Read the model definition and answer for the solid it produces. Units are mm, in the model's axes. Face numbers are marked on the shaded views. A direction names the side the tool comes from. Give positions to 0.01 mm unless a question says otherwise; leave off trailing zeros. Loops run counter-clockwise (first coordinate to the right, second up) from the corner with the lowest first, then second, coordinate; pieces in that order, holes last. Notation, with made-up numbers: (89, 34) - (140, 34) arc R23 ccw to (140, 58) - close; hole circle Ø1 at (-38.75, 37.25). An arc over 180 degrees is marked (long way). Put each result on its own line as item: value. Start each with the question number.
1. For the marked faces 1, 2, 3 and 4, determine the directions among +Z, -Z, +X, -X, +Y, -Y from which every point of the face is accessible in a straight line to the end or side of a thin tool.
2. A cutting plane is placed at A-A, the plane z = -4.5. Determine the outline of the cut face in (x, y).
3. A cutting plane is placed at B-B, the plane x = -27. Determine the outline of the cut face in (y, z).
4. A cutting plane is placed at D-D, the plane z = -10.5. Determine the outline of the cut face in (x, y), plus the area to 3 significant figures.
5. Consider L1, parallel to Z at x = -22.5, y = 1.7; L2, parallel to Y at x = -27, z = 6.05; L3, parallel to Z at x = -10, y = 3.9. Determine where each line is inside the solid, lowest interval first. Write a range as from..to.
6. Given pin 1 Ø1.9 at (x, y) = (-4, 3) entering from -Z; pin 2 Ø3 at (y, z) = (5, -3.5) entering from -X; pin 3 Ø2.5 at (y, z) = (2, 6) entering from -X; pin 4 Ø1.5 at (y, z) = (2.5, -10) entering from -X, each flat-ended and moving along its own axis, determine where each tip first touches the part or whether it passes through.
7. A cutting plane is placed at C-C, the plane x = -4. Determine the outline of the cut face in (y, z), plus the area to 3 significant figures.
8. For a pull along Z with two mould halves and no side action, classify the marked faces 5, 6, 7 and 8 as released by +Z, released by -Z, zero draft, split by the parting line, or undercut.
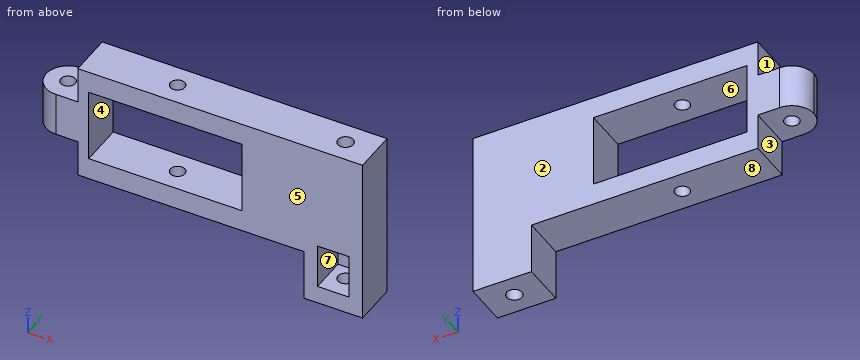
Autodesk Inventor part; units mm, degrees
ref_plane "Pracovní rovina1" through (0, 0, 0) normal (0, 0, -1) x (-1, 0, 0)
ref_plane "YZ Plane" through (0, 0, 0) normal (1, 0, 0) x (0, 1, 0)
ref_plane "XZ Plane" through (0, 0, 0) normal (0, 1, 0) x (-1, 0, 0)
sketch "Sketch1" plane through (0, 0, 0) normal (0, 1, 0) x (-1, 0, 0)
  line L0 (0, 0) -> (18.1846, 0) construction
  line L1 (0, 0) -> (0, 15)
  line L2 (0, 15) -> (8, 15)
  line L3 (8, 15) -> (8, 8)
  line L4 (8, 8) -> (39, 8)
  line L5 (39, 8) -> (39, 3)
  line L6 (39, 3) -> (45, 3)
  line L7 (45, 3) -> (45, 0)
  line L8 (0, 0) -> (0, -15)
  line L9 (0, -15) -> (8, -15)
  line L10 (8, -15) -> (8, -8)
  line L11 (8, -8) -> (39, -8)
  line L12 (39, -8) -> (39, -3)
  line L13 (39, -3) -> (45, -3)
  line L14 (45, -3) -> (45, 0)
  point P0 (45, 1.5)
  dimension "d0" = 6
  dimension "d1" = 45
  dimension "d2" = 8
  dimension "d3" = 8
  dimension "d4" = 15
  dimension "d5" = 3
extrude "Extrusion1" add sketch "Sketch1" along normal blind 6
sketch "Sketch2" plane through (-39, 0, -3) normal (0, 0, -1) x (-1, 0, 0)
  line L0 (0, 0) -> (6, 0)
  line L1 (6, 0) -> (6, 6)
  line L2 (0, 6) -> (6, 6)
  line L3 (0, 0) -> (0, 6)
  circle A0 centre (3, 3) radius 1
  point P0 (-39, 0)
  point P1 (6, 3)
  dimension "d8" = 3
  dimension "d9" = 2
extrude "Extrusion2" cut sketch "Sketch2" against normal blind 6 contours A0
sketch "Sketch3" plane through (0, 6, 0) normal (0, 1, 0) x (1, 0, 0)
  line L0 (-8, 15) -> (-8, 8)
  line L1 (-8, 8) -> (-39, 8)
  line L2 (-39, 8) -> (-39, 3)
  line L3 (-39, 3) -> (-45, 3)
  line L4 (-45, 3) -> (-45, -3)
  line L5 (-45, -3) -> (-39, -3)
  line L6 (-39, -3) -> (-39, -8)
  line L7 (-39, -8) -> (-8, -8)
  line L8 (-8, -8) -> (-8, -15)
  line L9 (-8, -15) -> (0, -15)
  line L10 (0, -15) -> (0, 15)
  line L11 (0, 15) -> (-8, 15)
  line L12 (-45, 3) -> (-45, -3) construction
  line L13 (-45, 0) -> (0, 0) construction
  line L14 (-16.5, -5) -> (-37.5, -5)
  line L15 (-37.5, -5) -> (-37.5, 5)
  line L16 (-37.5, 5) -> (-16.5, 5)
  line L17 (-16.5, 5) -> (-16.5, -5)
  point P0 (-42, -3)
  point P1 (-27, -5)
  dimension "d12" = 10
  dimension "d13" = 21
  dimension "d14" = 15
extrude "Extrusion3" cut sketch "Sketch3" against normal through all contours L14 L15 L16 L17
sketch "Sketch4" plane through (-8, 0, -8) normal (0, 0, -1) x (-1, 0, 0)
  line L0 (29.5, 0) -> (8.5, 0)
  line L1 (29.5, 6) -> (29.5, 0)
  line L2 (8.5, 6) -> (29.5, 6)
  line L3 (8.5, 6) -> (8.5, 0)
  circle A0 centre (19, 3) radius 1
  point P0 (-8, 0)
  point P1 (10.5, 6)
  point P2 (29.5, 3)
  point P3 (19, 6)
  dimension "d17" = 2
extrude "Extrusion4" cut sketch "Sketch4" against normal through all contours A0
fillet "Fillet1" radius 3 2 edges at (-45, 6, 0) (-45, 0, 0)
sketch "Náčrt5" plane through (0, 0, -15) normal (0, 0, -1) x (-1, 0, 0)
  line L0 (0, 0) -> (8, 0)
  line L1 (8, 0) -> (8, 6)
  line L2 (0, 6) -> (8, 6)
  line L3 (0, 0) -> (0, 6)
  circle A0 centre (4, 3) radius 1.05
  point P0 (0, 0)
  point P1 (8, 3)
  point P2 (4, 6)
  dimension "d21" = 2.1
extrude "Vysunutí5" cut sketch "Náčrt5" against normal through all contours A0
ref_plane "Pracovní rovina1" through (0, 0, 0) normal (0, 0, -1) x (-1, 0, 0)
sketch "Sketch9" plane through (0, 0, 0) normal (0, -1, 0) x (1, 0, 0)
  line L0 (-42, -3) -> (-42, 3)
  line L1 (-39, -3) -> (-42, -3)
  line L2 (-39, -8) -> (-39, -3)
  line L3 (-8, -8) -> (-39, -8)
  line L4 (-8, -15) -> (-8, -8)
  line L5 (0, -15) -> (-8, -15)
  line L6 (0, 15) -> (0, -15)
  line L7 (-8, 15) -> (0, 15)
  line L8 (-8, 8) -> (-8, 15)
  line L9 (-39, 8) -> (-8, 8)
  line L10 (-39, 3) -> (-39, 8)
  line L11 (-42, 3) -> (-39, 3)
  line L12 (-16.5, -5) -> (-37.5, -5)
  line L13 (-37.5, -5) -> (-37.5, 5)
  line L14 (-37.5, 5) -> (-16.5, 5)
  line L15 (-16.5, 5) -> (-16.5, -5)
  line L16 (-2.95, -15) -> (-5.05, -15)
  line L17 (-1.8376, -6.4564) -> (-6.1624, -6.4564)
  line L18 (-6.1624, -6.4564) -> (-6.1624, -12.5436)
  line L19 (-6.1624, -12.5436) -> (-1.8376, -12.5436)
  line L20 (-1.8376, -12.5436) -> (-1.8376, -6.4564)
  line L21 (0, -15) -> (-8, -15) construction
  line L22 (-4, -15) -> (-4, 15) construction
  line L23 (-8, 15) -> (0, 15) construction
  point P0 (0, 0)
  point P1 (0, 0)
  point P2 (-1.8376, -9.5)
  dimension "d29" = 9.5
extrude "Extrusion7" cut sketch "Sketch9" against normal blind 5 contours L20 L19 L18 L17
sketch "Sketch10" plane through (0, 0, 0) normal (0, -1, 0) x (1, 0, 0)
  line L0 (-1.8376, -12.5436) -> (-6.1624, -12.5436)
  line L1 (-6.1624, -12.5436) -> (-6.1624, -6.4564)
  line L2 (-6.1624, -6.4564) -> (-1.8376, -6.4564)
  line L3 (-1.8376, -6.4564) -> (-1.8376, -12.5436)
  line L4 (-42, -3) -> (-42, 3)
  line L5 (-39, -3) -> (-42, -3)
  line L6 (-39, -8) -> (-39, -3)
  line L7 (-8, -8) -> (-39, -8)
  line L8 (-8, -15) -> (-8, -8)
  line L9 (0, -15) -> (-8, -15)
  line L10 (0, 15) -> (0, -15)
  line L11 (-8, 15) -> (0, 15)
  line L12 (-8, 8) -> (-8, 15)
  line L13 (-39, 8) -> (-8, 8)
  line L14 (-39, 3) -> (-39, 8)
  line L15 (-42, 3) -> (-39, 3)
  line L16 (-37.5, -5) -> (-37.5, 5)
  line L17 (-37.5, 5) -> (-16.5, 5)
  line L18 (-16.5, 5) -> (-16.5, -5)
  line L19 (-16.5, -5) -> (-37.5, -5)
  line L20 (-8, 8) -> (-8, 15)
  line L21 (-8, 8) -> (0, 8)
  point P0 (0, 0)
extrude "Extrusion8" cut sketch "Sketch10" against normal through all contours L12 L11 L10 L21
properties part number "drzak_pritlacneho_kolecka"
Return value:
1. face 1: +Z, -X, +Y, -Y
1. face 2: +Z, -Z, +X, -X, +Y
1. face 3: -Z, -X, +Y, -Y
1. face 4: +Y, -Y
2. outline: (-39, 0) - (-37.5, 0) - (-37.5, 6) - (-39, 6) - close; (-16.5, 0) - (0, 0) - (0, 6) - (-16.5, 6) - close; hole circle Ø2.1 at (-4, 3)
3. outline: (0, -8) - (2, -8) - (2, -5) - (0, -5) - close; (0, 5) - (2, 5) - (2, 8) - (0, 8) - close; (4, -8) - (6, -8) - (6, -5) - (4, -5) - close; (4, 5) - (6, 5) - (6, 8) - (4, 8) - close
4. outline: (-8, 0) - (-6.16, 0) - (-6.16, 5) - (-1.84, 5) - (-1.84, 0) - (0, 0) - (0, 6) - (-8, 6) - close
4. area: 26.4 mm2
5. L1: z = -8..-5, 5..8
5. L2: y = 0..2, 4..6
5. L3: z = -8..8
6. pin 1: passes through
6. pin 2: stops at x = -44.94
6. pin 3: stops at x = -39
6. pin 4: stops at x = -8
7. outline: (0, -15) - (1.95, -15) - (1.95, -12.54) - (0, -12.54) - close; (0, -6.46) - (1.95, -6.46) - (1.95, 8) - (0, 8) - close; (4.05, -15) - (6, -15) - (6, 8) - (4.05, 8) - (4.05, -6.46) - (5, -6.46) - (5, -12.54) - (4.05, -12.54) - close
7. area: 72.0 mm2
8. face 5: zero draft
8. face 6: undercut
8. face 7: undercut
8. face 8: released by -Z
